Design review of the part built by this model. Coordinates are the model's own, in mm. A direction names the side the tool comes from. Give positions to 0.01 mm unless a question says otherwise; leave off trailing zeros. Order: outer loops, then holes, each group sorted by start corner. A loop starts at its lowest first (then second) coordinate and runs counter-clockwise, first axis right, second up. Notation, with made-up numbers: M 14.5,51.5 L 61.5,51.5 A20 cw 61.5,71.5 Z; hole C -11.75,-8 d7. An arc over 180 degrees is marked long. Answer as a JSON object with one key per item and string values.
from build123d import *

# Parameters (mm, degrees)
F0_W     = 84
F0_H     = 59
F1_DEPTH = 10.2
F2_W     = 87.5051617622
F2_H     = 61.1030906439
F2_W_2   = 3.5238564014
F3_DEPTH = 5
F4_W     = 5.2764372826
F4_H     = 61.1030906439
F5_DEPTH = 33.6
F7_DEPTH = 69.2
F8_R     = 2
F9_DEPTH = 12.1


with BuildPart() as f1:
    # F0 (on Front) → F1 (new body)
    with BuildSketch(Plane.XZ):
        Rectangle(F0_W, F0_H)
    extrude(amount=F1_DEPTH)

    # F2 (on face) → F3 (join)
    with BuildSketch(Plane(origin=(0, 0, 0), x_dir=(-1, 0, 0), z_dir=(0, 1, 0))):
        Rectangle(F2_W, F2_H)
        with Locations((45.5145090818, 0)):
            Rectangle(F2_W_2, F2_H)
    extrude(amount=F3_DEPTH)

    # F4 (on face) → F5 (join)
    with BuildSketch(Plane.XZ):
        with Locations((-44.6382186413, 0)):
            Rectangle(F4_W, F4_H)
    extrude(amount=F5_DEPTH)

    # F6 (on face) → F7 (cut)
    with BuildSketch(Plane(origin=(0, 0, -30.5515453219), x_dir=(1, 0, 0), z_dir=(0, 0, -1))):
        with BuildLine():
            ThreePointArc((-45.8268001676, 33.6), (-43.1548823666, 24.5698804652), (-42, 15.2238411829))
            Line((-42, 15.2238411829), (-42, 33.6))
            Line((-42, 33.6), (-45.8268001676, 33.6))
        make_face()
    extrude(amount=-F7_DEPTH, mode=Mode.SUBTRACT)

    # F8 (on face) → F9 (join)
    with BuildSketch(Plane(origin=(0, 5, 0), x_dir=(-1, 0, 0), z_dir=(0, 1, 0))):
        with Locations((-33.7525808811, 20.5515453219)):
            Circle(F8_R)
        with Locations((37.2764372826, 20.5515453219)):
            Circle(F8_R)
        with Locations((37.2764372826, -20.5515453219)):
            Circle(F8_R)
        with Locations((-33.7525808811, -20.5515453219)):
            Circle(F8_R)
    extrude(amount=F9_DEPTH)


solid = f1.part
(1) Tool access review of faces 4 (the flat face through (-1, -5, 29.5)), 5 (the cylindrical face through (-37.02, 10.97, -18.57)), 6 (the flat face through (-1, -10.2, 0)): name each direction out of +Z, -Z, +X, -X, +Y, -Y from which nothing blocks a thin tool from reaching the whole face with its end or side.
Checked values:
{"face 4": "+Z, +X, -Y", "face 5": "+Y", "face 6": "+Z, -Z, +X, -Y"}
(2) We need section D-D (y = 7). Write out the cut boundary in (x, z), plus the area to 3 significant figures.
Checked values:
{"outline": "C -37.28,-20.55 d4; C -37.28,20.55 d4; C 33.75,-20.55 d4; C 33.75,20.55 d4", "area": "50.3 mm^2"}
(3) We need section C-C (z = 26). Write out the cut boundary in (x, y).
Checked values:
{"outline": "M -47.28,-33.6 L -45.83,-33.6 A57.23 ccw -42,-15.22 L -42,-10.2 L 42,-10.2 L 42,0 L 43.75,0 L 43.75,5 L -47.28,5 Z"}
(4) Insertion check: pin 1 (8 mm diameter, centred on x = 26, z = 20, fed in from +Y); pin 2 (7.5 mm diameter, centred on y = -9.5, z = -4, fed in from +X); pin 3 (5 mm diameter, centred on x = 5.5, y = -6.5, fed in from -Z). Each pin has a flat end and moves straight along its axis. Give the tip position at first contact, or say it passes through.
Checked values:
{"pin 1": "stops at y = 5", "pin 2": "stops at x = 42", "pin 3": "stops at z = -29.5"}
(5) Draft analysis for pull direction Z (two halves, no side actions). For faces 1 (the flat face through (42, -5, 0)), 2 (the flat face through (-1, -5, -29.5)), 3 (the cylindrical face through (35.75, 10.97, 20.64)), state which applies: +Z half, -Z half, draft (parallel to the pull), parting line (faces both ways), or undercut.
Checked values:
{"face 1": "draft", "face 2": "-Z half", "face 3": "undercut"}
(6) To check wall thickness, follow L1, parallel to X at y = -15, z = 1; L2, parallel to Y at x = -26, z = 25.5; L3, parallel to Z at x = 23.5, y = -6. State the ranges of each line that lie inside material, in increasing order. Write a range as from..to.
Checked values:
{"L1": "x = -47.28..-42", "L2": "y = -10.2..5", "L3": "z = -29.5..29.5"}
(7) We need section B-B (y = -3.5). Write out the cut boundary in (x, z), plus the area to 3 significant figures.
Checked values:
{"outline": "M -47.28,-30.55 L -42,-30.55 L -42,-29.5 L 42,-29.5 L 42,29.5 L -42,29.5 L -42,30.55 L -47.28,30.55 Z", "area": "5,280 mm^2"}
(8) We need section A-A (x = -22.5). Write out the cut boundary in (y, z).
Checked values:
{"outline": "M -10.2,-29.5 L 0,-29.5 L 0,-30.55 L 5,-30.55 L 5,30.55 L 0,30.55 L 0,29.5 L -10.2,29.5 Z"}
